Can you work these out from the model? Positions are in its coordinate system, mm. Face numbers are marked on the shaded views. A direction names the side the tool comes from. Coordinates: 2 decimals unless noted, no trailing zeros. Order: outer loops, then holes, each group sorted by start corner. A loop starts at its lowest first (then second) coordinate and runs counter-clockwise, first axis right, second up.
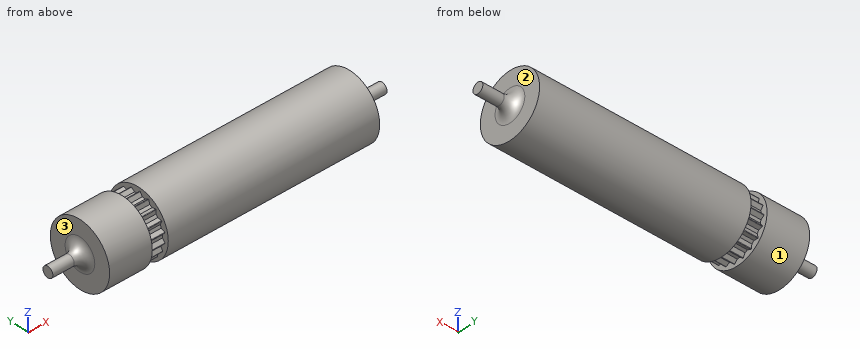
```python
from build123d import *

# Parameters (mm, degrees)
CONG_1_R                     = 5
BOSS_EXTRU_1_DEPTH           = 7.5
R_P_TITION_CIRCULAIRE1_COUNT = 19


with BuildPart() as part:
    # Esquisse1 → Révolution1 (revolve)
    with BuildSketch(Plane.XY, mode=Mode.PRIVATE) as r_volution1_sk:
        Polygon((-78.3, 0), (-78.3, 2.5), (-63.3, 2.5), (-63.3, 15), (-43.3, 15), (-43.3, 12), (-35.8, 12), (-35.8, 15), (63.3, 15), (63.3, 2.5), (78.3, 2.5), (78.3, 0), align=None)
    revolve(r_volution1_sk.sketch.rotate(Axis((-78.3, 0, 0), (1, 0, 0)), 180), axis=Axis((-78.3, 0, 0), (1, 0, 0)))

    # Congé1
    cong_1_edges = [part.edges().sort_by_distance(p)[0] for p in [
        (63.3, 2.5, 0),
        (-63.3, 2.5, 0),
    ]]
    fillet(cong_1_edges, radius=CONG_1_R)

    # Esquisse3 → Boss.-Extru.1 (add)
    with BuildSketch(Plane(origin=(-43.3, 0, 0), x_dir=(0, 0, -1), z_dir=(1, 0, 0))):
        with BuildLine():
            Line((0.601733572, 13.451614371), (2.134408168, 11.226678946))
            Line((2.134408168, 11.226678946), (-1.394925929, 11.342318989))
            Line((-1.394925929, 11.342318989), (0.280106761, 13.462152602))
            ThreePointArc((0.280106761, 13.462152602), (0.443579587, 13.538049), (0.601733572, 13.451614371))
        make_face()
    boss_extru_1 = extrude(amount=BOSS_EXTRU_1_DEPTH)

    # Répétition circulaire1: Boss.-Extru.1 ×19 about axis
    r_p_tition_circulaire1_axis = Axis((0, 0, 0), (1, 0, 0))
    for i in range(1, R_P_TITION_CIRCULAIRE1_COUNT):
        add(boss_extru_1.rotate(r_p_tition_circulaire1_axis, i * 360 / R_P_TITION_CIRCULAIRE1_COUNT))


solid = part.part
```
1. Imagine slicing it at B-B on x = -66.5. Please give me the cut outline in (y, z), then the cut area to 3 significant figures.
Completed:
outline: circle Ø5.67 at (0, 0)
area: 25.3 mm2
2. Imagine slicing it at A-A on x = 25. Please give me the cut outline in (y, z), then the cut area to 3 significant figures.
Completed:
outline: circle Ø30 at (0, 0)
area: 707 mm2
3. I'm going to push flat-ended pins straight in: pin 1 (1 mm diameter, centred on x = 44, z = 8, fed in from +Y); pin 2 (4 mm diameter, centred on y = -11.5, z = -3.5, fed in from +X); pin 3 (12 mm diameter, centred on y = -2.5, z = 8.5, fed in from -X). Where does each tip first touch, or does it pass through?
Completed:
pin 1: stops at y = 12.99
pin 2: stops at x = 63.3
pin 3: stops at x = -66.44
4. Please list where these lines run through material, in increasing order: probe 1 along X at (y, z) = (-6, 11.5); probe 2 along X at (y, z) = (8, -1.5); probe 3 along Z at (x, y) = (59, -11.5).
Completed:
probe 1: x = -63.3 to -43.3, -35.8 to 63.3
probe 2: x = -63.3 to 63.3
probe 3: z = -9.63 to 9.63
5. On a 3-axis mill with a long thin cutter (end or side, diameter ignored), from which of +Z, -Z, +X, -X, +Y, -Y can I reach the whole of each face in a straight line? I mean the marked faces 1, 2 and 3. Say none if no direction works.
Completed:
face 1: +X, -X
face 2: +X
face 3: -X
